Can you work these out from the model? Positions are in its coordinate system, mm. Face numbers are marked on the shaded views. A direction names the side the tool comes from. Give positions to 0.01 mm unless a question says otherwise; leave off trailing zeros. Order: outer loops, then holes, each group sorted by start corner. A loop starts at its lowest first (then second) coordinate and runs counter-clockwise, first axis right, second up. Notation, with made-up numbers: M 85.25,84 L 123.25,84 A32 ccw 123.25,112 Z; hole C 10.5,-24.75 d1. An arc over 180 degrees is marked long. One line per question, with ' | ' between items. Start each with the question number.
1) If we section it at C-C, the plane x = -6: Please give me the cut outline in (y, z).
2) If we section it at B-B, the plane z = 8: Please give me the cut outline in (x, y), plus the area to 3 significant figures.
3) I'm going to push flat-ended pins straight in: pin 1 Ø1.3 at (x, z) = (-3, -3) entering from +Y; pin 2 Ø4 at (x, y) = (-4.5, 5) entering from -Z; pin 3 Ø5 at (x, z) = (-12.5, 9) entering from -Y. Where does each tip first touch, or does it pass through?
4) Please list where these lines run through material, in increasing order: line 1 along X through (y, z) = (15.5, 0); line 2 along Y through (x, z) = (9, -10.5). Write a range as [from, to].
5) Thinking about a two-plate mould opening in Z: for the marked faces 1, 2 and 3, which applies, +Z half, -Z half, draft (parallel to the pull), parting line (faces both ways), or undercut?
6) If we section it at D-D, the plane y = 10.75: Please give me the cut outline in (x, z).
7) If we section it at A-A, the plane z = -6: Please give me the cut outline in (x, y).
8) For the marked faces 4 and 5, which set-ups out of +Z, -Z, +X, -X, +Y, -Y let a thin tool reach every point of the face, with its end or its side?
Autodesk Inventor part; units mm, degrees
ref_plane "YZ Plane" through (0, 0, 0) normal (1, 0, 0) x (0, 1, 0)
ref_plane "XZ Plane" through (0, 0, 0) normal (0, 1, 0) x (-1, 0, 0)
ref_plane "XY Plane" through (0, 0, 0) normal (0, 0, 1) x (1, 0, 0)
sketch "스케치1" plane through (0, 0, 0) normal (0, 1, 0) x (-1, 0, 0)
  circle A0 centre (0, 0) radius 5
  dimension "d0" = 10
extrude "돌출1" add sketch "스케치1" along normal blind 15
sketch "스케치2" plane through (0, 15, 0) normal (0, 1, 0) x (1, 0, 0)
  circle A0 centre (0, 0) radius 15
  circle A1 centre (0, 0) radius 16
  dimension "d3" = 30
  dimension "d4" = 32
extrude "돌출2" add sketch "스케치2" along normal blind 1.5
sketch "스케치3" plane through (0, 15, 0) normal (0, 1, 0) x (1, 0, 0)
  line L0 (0, 0) -> (15, 0)
  circle A0 centre (0, 0) radius 15
  line L1 (0, 0) -> (14.4889, 3.8823)
  line L2 (0, 0) -> (15, 0) construction
  line L3 (0, 0) -> (12.9904, 7.5)
  line L4 (0, 0) -> (15, 0) construction
  line L5 (0, 0) -> (10.6066, 10.6066)
  line L6 (0, 0) -> (15, 0) construction
  line L7 (0, 0) -> (7.5, 12.9904)
  line L8 (0, 0) -> (15, 0) construction
  line L9 (0, 0) -> (3.8823, 14.4889)
  line L10 (0, 0) -> (15, 0) construction
  line L11 (0, 0) -> (0, 15)
  line L12 (0, 0) -> (-3.8823, 14.4889)
  line L13 (0, 0) -> (-7.5, 12.9904)
  line L14 (0, 0) -> (-10.6066, 10.6066)
  line L15 (0, 0) -> (-12.9904, 7.5)
  line L16 (0, 0) -> (-14.2878, 3.8284)
  line L17 (0, 0) -> (-12.9904, -7.5)
  line L18 (0, 0) -> (-7.5, -12.9904)
  line L19 (0, 0) -> (0, -15)
  line L20 (0, 0) -> (10.6066, -10.6066)
  line L21 (0, 0) -> (12.9904, -7.5)
  line L22 (0, 0) -> (14.4889, -3.8823)
  line L23 (0, 0) -> (-15, 0)
  line L24 (0, 0) -> (-14.4889, -3.8823)
  line L25 (0, 0) -> (0, 0)
  line L26 (0, 0) -> (-10.6066, -10.6066)
  line L27 (0, 0) -> (-3.8823, -14.4889)
  line L28 (0, 0) -> (7.5, -12.9904)
  line L29 (0, 0) -> (3.8823, -14.4889)
  line L30 (0, 0) -> (-14.4889, 3.8823)
  dimension "d12" = 15
  dimension "d13" = 15
  dimension "d14" = 15
  dimension "d15" = 15
  dimension "d16" = 15
  dimension "d17" = 15
  dimension "d18" = 15
  dimension "d19" = 15
  dimension "d21" = 15
  dimension "d22" = 15
  dimension "d23" = 15
  dimension "d24" = 15
  dimension "d25" = 15
  dimension "d26" = 15
  dimension "d27" = 15
  dimension "d28" = 15
  dimension "d29" = 15
  dimension "d30" = 15
  dimension "d31" = 15
  dimension "d32" = 15
  dimension "d33" = 15
  dimension "d34" = 15
  dimension "d35" = 15
  dimension "d36" = 15
  dimension "d7" = 15
  dimension "d8" = 30
  dimension "d9" = 45
  dimension "d10" = 60
  dimension "d11" = 75
  dimension "d20" = 15
extrude "돌출3" add sketch "스케치3" along normal blind 0.2 contours L3 A0 L1 | L7 A0 L5 | L11 A0 L9 | L13 A0 L12 | L15 A0 L14 | L23 A0 L30 L16 | L21 A0 L20 | L0 A0 L22 | L17 A0 L24 | L18 A0 L26 | L19 A0 L27 | L28 A0 L29
sketch "스케치4" plane through (0, 16.5, 0) normal (0, 1, 0) x (1, 0, 0)
  line L0 (0, 0) -> (10.6066, 10.6066)
  circle A0 centre (0, 0) radius 2
  line L1 (0, 0) -> (14.4889, 3.8823)
  circle A1 centre (0, 0) radius 1
  dimension "d39" = 4
  dimension "d40" = 2
extrude "돌출4" add sketch "스케치4" against normal blind 2 contours A1 L1 A0 L0 | L0 A0 L1 A1
sketch "스케치5" plane through (0, 16.5, 0) normal (0, 1, 0) x (1, 0, 0)
  point P0 (0, 0)
properties part number "fan_num3"
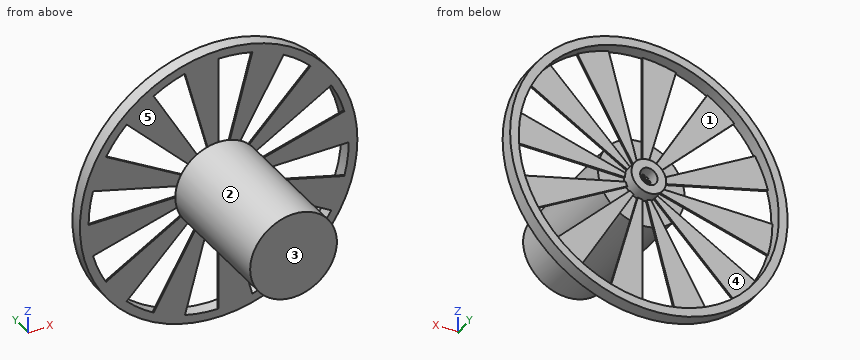
Results found:
1) outline: M 15,-14.83 L 16.5,-14.83 L 16.5,-13.75 L 15.2,-13.75 L 15.2,-10.39 L 15,-10.39 Z; M 15,-6 L 15.2,-6 L 15.2,-3.46 L 15,-3.46 Z; M 15,-1.61 L 15.2,-1.61 L 15.2,0 L 15,0 Z; M 15,1.61 L 15.2,1.61 L 15.2,3.46 L 15,3.46 Z; M 15,6 L 15.2,6 L 15.2,10.39 L 15,10.39 Z; M 15,13.75 L 16.5,13.75 L 16.5,14.83 L 15,14.83 Z
2) outline: M -13.86,15 L -12.69,15 L -12.69,16.5 L -13.86,16.5 Z; M -8,15 L -4.62,15 L -4.62,15.2 L -8,15.2 Z; M -2.14,15 L 0,15 L 0,15.2 L -2.14,15.2 Z; M 2.14,15 L 4.62,15 L 4.62,15.2 L 2.14,15.2 Z; M 8,15 L 13.86,15 L 13.86,16.5 L 12.69,16.5 L 12.69,15.2 L 8,15.2 Z | area: 6.04 mm²
3) pin 1: stops at y = 15.2 | pin 2: stops at z = -4.33 | pin 3: stops at y = 15
4) line 1: x = [-16, -15], [-2, -1], [1, 2], [15, 16] | line 2: y = [15, 15.2]
5) face 1: undercut | face 2: parting line | face 3: draft
6) outline: C 0,0 d10
7) outline: M -14.83,15 L -13.75,15 L -13.75,16.5 L -14.83,16.5 Z; M -10.39,15 L -6,15 L -6,15.2 L -10.39,15.2 Z; M -3.46,15 L -1.61,15 L -1.61,15.2 L -3.46,15.2 Z; M 0,15 L 1.61,15 L 1.61,15.2 L 0,15.2 Z; M 3.46,15 L 6,15 L 6,15.2 L 3.46,15.2 Z; M 10.39,15 L 14.83,15 L 14.83,16.5 L 13.75,16.5 L 13.75,15.2 L 10.39,15.2 Z
8) face 4: +Y | face 5: -Y
